CAD build for the part. Positions are in the model's coordinates, mm. Face numbers are marked on the shaded views. A direction names the side the tool comes from. Coordinates: 2 decimals unless noted, no trailing zeros. Loops run counter-clockwise (first coordinate to the right, second up) from the corner with the lowest first, then second, coordinate; pieces in that order, holes last.
1) Saw through at C-C, the plane x = 4. Write the cut outline in (y, z).
2) Two-plate mould, pull along X, no slides. Class the marked faces 4, 5 and 6: +X half, -X half, draft (parallel to the pull), parting line (faces both ways), or undercut.
3) Saw through at B-B, the plane z = 0.3. Write the cut outline in (x, y).
4) Which spindle directions (+Z, -Z, +X, -X, +Y, -Y) get a long thin tool onto all of the face, cutting with end or side? Do the marked faces 1, 2 and 3. Say none if no direction does.
5) Wall check: line 1 along X through (y, z) = (4.5, 0.65); line 2 along Y through (x, z) = (-2, 1.2); line 3 along X through (y, z) = (-3.75, 1.15). Give the ranges that are in metal, low to high.
6) Saw through at D-D, the plane z = 2. Write the cut outline in (x, y).
7) Pin check, flat tips, straight feed: pin 1 Ø8 at (x, y) = (5, 4.5) entering from +Z; pin 2 Ø1.6 at (x, y) = (7, -0.5) entering from +Z. Stop position of each tip, or through.
8) Saw through at A-A, the plane y = 0.75. Write the cut outline in (x, z).
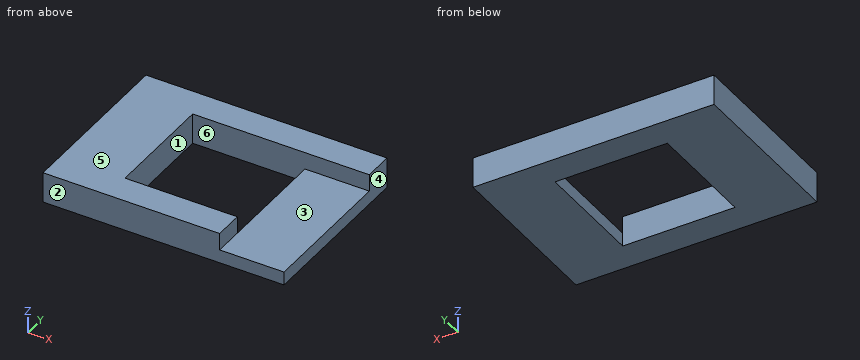
```python
from build123d import *

# Parameters (mm, degrees)
F0_W     = 19.742636
F0_H     = 14
F0_W_2   = 9.2
F0_H_2   = 9.2
F1_DEPTH = 2.5
F2_W     = 10
F2_H     = 20
F3_DEPTH = 1.4


with BuildPart() as f1:
    # F0 (on Top) → F1 (new body)
    with BuildSketch(Plane.XY):
        Rectangle(F0_W, F0_H)
        Rectangle(F0_W_2, F0_H_2, mode=Mode.SUBTRACT)
    extrude(amount=F1_DEPTH)

    # F2 (on face) → F3 (cut)
    with BuildSketch(Plane.XY.offset(2.5)):
        with Locations((9.6, -5.4)):
            Rectangle(F2_W, F2_H)
    extrude(amount=-F3_DEPTH, mode=Mode.SUBTRACT)


solid = f1.part
```
Data:
1. outline: (-7, 0) - (-4.6, 0) - (-4.6, 2.5) - (-7, 2.5) - close; (4.6, 0) - (7, 0) - (7, 2.5) - (4.6, 2.5) - close
2. face 4: +X half
2. face 5: draft
2. face 6: undercut
3. outline: (-9.87, -7) - (9.87, -7) - (9.87, 7) - (-9.87, 7) - close; hole (-4.6, -4.6) - (4.6, -4.6) - (4.6, 4.6) - (-4.6, 4.6) - close
4. face 1: +Z, -Z
4. face 2: +Z, -Z, +X, -X, -Y
4. face 3: +Z, +X, -Y
5. line 1: x = -9.87 to -4.6, 4.6 to 9.87
5. line 2: y = -7 to -4.6, 4.6 to 7
5. line 3: x = -9.87 to -4.6
6. outline: (-9.87, -7) - (4.6, -7) - (4.6, -4.6) - (-4.6, -4.6) - (-4.6, 4.6) - (9.87, 4.6) - (9.87, 7) - (-9.87, 7) - close
7. pin 1: stops at z = 2.5
7. pin 2: stops at z = 1.1
8. outline: (-9.87, 0) - (-4.6, 0) - (-4.6, 2.5) - (-9.87, 2.5) - close; (4.6, 0) - (9.87, 0) - (9.87, 1.1) - (4.6, 1.1) - close
